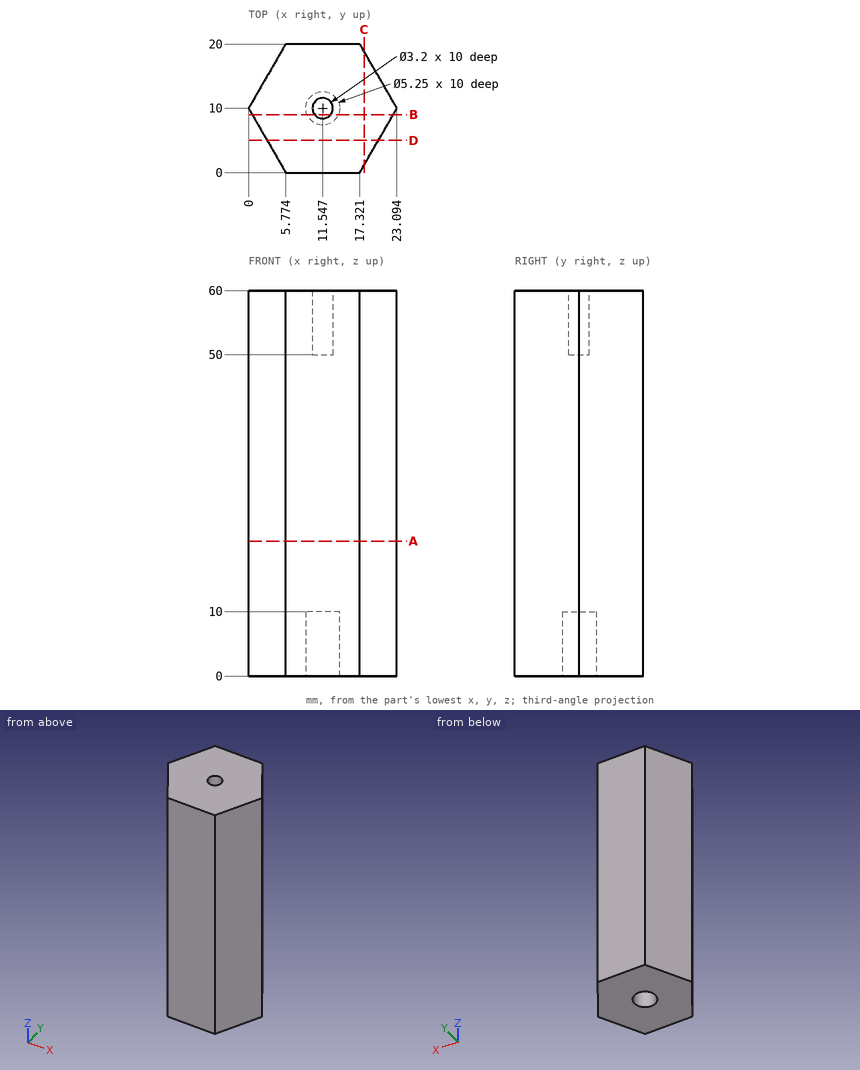
Answer from the drawing. Dimensions are ordinates in mm from the lowest x, y and z of the part. Coordinates: 2 decimals unless noted, no trailing zeros. Write each loop counter-clockwise with the first axis right and the second up, starting at its lowest first coordinate (ties: lowest second). Pieces come first, ordered by that corner, then holes. Notation, with made-up numbers: M 1.5,-39 L 45.5,-39 A13 cw 45.5,-17 Z; hole C 67,8.5 d9. An arc over 180 degrees is marked long. Use one line per item in the form item = value. Start each with the question number.
1. The part is cut by section B-B (y = 9). Give the vertices of the cut face in (x, z) (1 decimal).
2. The part is cut by section A-A (z = 21). Give the vertices of the cut face in (x, y) (1 decimal), plus the area to 3 significant figures.
3. The part is cut by section C-C (x = 18). Give the vertices of the cut face in (y, z), plus the area to 3 significant figures.
4. Each of these flat-tipped pins is pushed along its axis until it touches: P1, Ø10, axis at y = 17.5, z = 7.5, coming from the +X side; P2, Ø1, axis at x = 11, y = 10.5, coming from the +Z side; P3, Ø4, axis at x = 3, z = 18, coming from the -Y side. Where does it stop, or does it pass through?
5. Straight lines are drawn through the part: probe 1 along Z at (x, y) = (10, 8.5); probe 2 along Y at (x, z) = (2, 54) (1 decimal); probe 3 along X at (y, z) = (12.75, 31) (1 decimal). For each, find the intervals that lie inside material, in ascending order. Write a range as from..to.
6. The part is cut by section D-D (y = 5). Give the vertices of the cut face in (x, z), plus the area to 3 significant figures.
Evaluation:
q1.outline = M 0.6,0 L 9.1,0 L 9.1,10 L 14,10 L 14,0 L 22.5,0 L 22.5,60 L 12.8,60 L 12.8,50 L 10.3,50 L 10.3,60 L 0.6,60 Z
q2.outline = M 0,10 L 5.8,0 L 17.3,0 L 23.1,10 L 17.3,20 L 5.8,20 Z
q2.area = 346 mm^2
q3.outline = M 1.18,0 L 18.82,0 L 18.82,60 L 1.18,60 Z
q3.area = 1,060 mm^2
q4.P1 = 21.65
q4.P2 = 50
q4.P3 = 1.34
q5.probe_1 = 10..60
q5.probe_2 = 6.5..13.5
q5.probe_3 = 1.6..21.5
q6.outline = M 2.89,0 L 20.21,0 L 20.21,60 L 2.89,60 Z
q6.area = 1,040 mm^2
